Autodesk Inventor part; units mm, degrees
ref_plane "YZ Plane" through (0, 0, 0) normal (1, 0, 0) x (0, 1, 0)
ref_plane "XZ Plane" through (0, 0, 0) normal (0, 1, 0) x (-1, 0, 0)
ref_plane "XY Plane" through (0, 0, 0) normal (0, 0, 1) x (1, 0, 0)
sketch "Náčrt1" plane through (0, 0, 0) normal (0, 0, 1) x (1, 0, 0)
  line L0 (-9.5, 7.7937) -> (-9.5, -1.7063)
  line L1 (-9.5, -1.7063) -> (9.5, -1.7063)
  line L2 (9.5, -1.7063) -> (9.5, 7.7937)
  line L3 (9.5, 7.7937) -> (10, 7.7937)
  line L4 (10, 7.7937) -> (10, -2.2063)
  line L5 (10, -2.2063) -> (-10, -2.2063)
  line L6 (-10, -2.2063) -> (-10, 7.7937)
  line L7 (-10, 7.7937) -> (-9.5, 7.7937)
  point P0 (0, 0)
  point P1 (9.5, 3.0437)
  point P2 (-9.75, 7.7937)
  point P3 (9.75, 7.7937)
  dimension "d0" = 10
  dimension "d1" = 10
  dimension "d2" = 0.5
  dimension "d3" = 0.5
  dimension "d4" = 0.5
  dimension "d5" = 10
  dimension "d6" = 10
extrude "Vysunutí1" add sketch "Náčrt1" along normal blind 10
sketch "Náčrt2" plane through (10, -2.2063, 0) normal (1, 0, 0) x (0, 0, -1)
  circle A0 centre (-5, 5) radius 2
  line L0 (0, 0) -> (0, 10)
  point P0 (0, 2.2063)
  point P1 (0, 5)
  dimension "d9" = 4
  dimension "d10" = 5
extrude "Vysunutí2" cut sketch "Náčrt2" against normal through all
pattern_linear "Obdélníkové pole1" count 10 spacing 10 along (0, 0, 1) of "Vysunutí2"
sketch "Náčrt3" plane through (-9.5, -1.7063, 0) normal (0, 1, 0) x (1, 0, 0)
  circle A0 centre (4.5, -5) radius 2
  line L0 (19, -10) -> (0, -10)
  line L1 (-0.5, 0) -> (-0.5, -10)
  point P0 (9.5, 0)
  dimension "d16" = 4
  dimension "d17" = 5
  dimension "d18" = 5
extrude "Vysunutí3" cut sketch "Náčrt3" against normal through all
pattern_linear "Obdélníkové pole2" count 10 spacing 10 along (0, 0, -1) count 5 spacing 10 along (1, 0, 0) of "Vysunutí3"
sketch "Náčrt4" plane through (10, -2.2063, 0) normal (1, 0, 0) x (0, 0, -1)
  arc A0 (0, 5) -> (-10, 5) centre (-5, 5) ccw
  line L0 (0, 0) -> (0, 10)
  line L1 (0, 0) -> (-10, 0)
  line L2 (0, 10) -> (-10, 10)
  line L3 (-10, 10) -> (0, 10)
  line L4 (0, 10) -> (0, 5)
  line L5 (0, 10) -> (0, 0.5)
  line L6 (-10, 10) -> (-10, 0.5)
  line L7 (-10, 5) -> (-10, 10)
  point P0 (0, 2.2063)
  point P1 (-5, 10)
  dimension "d27" = 10
  dimension "d28" = 5
  dimension "d29" = 5
extrude "Vysunutí4" cut sketch "Náčrt4" against normal through all
fillet "Zaoblení1" radius 0.5 2 edges at (10, -2.2063, 5) (9.5, -1.7063, 5)
fillet "Zaoblení2" radius 0.5 2 edges at (-10, -2.2063, 5) (-9.5, -1.7063, 5)
properties part number "4031"
Can you work these out from the model? Positions are in its coordinate system, mm. A direction names the side the tool comes from. Coordinates: 2 decimals unless noted, no trailing zeros. Order: outer loops, then holes, each group sorted by start corner. A loop starts at its lowest first (then second) coordinate and runs counter-clockwise, first axis right, second up. Notation, with made-up numbers: M 72,80.25 L 125,80.25 A27 ccw 125,113.25 Z; hole C -3.75,56.25 d8. An arc over 180 degrees is marked long. Write item = value, one per line.
(1) Suppose I cut it at B-B on x = 5. Please give me the cut outline in (y, z).
Results are:
outline = M -2.21,0 L -1.71,0 L -1.71,3 L -2.21,3 Z; M -2.21,7 L -1.71,7 L -1.71,10 L -2.21,10 Z
(2) For pin 1 Ø3 at (x, z) = (-5, 5) entering from -Y, with a flat end and sliding along its axis, tell me the tip position at first contact or that it passes through.
Results are:
pin_1 = through
(3) For faces 1 (the face through (0, -1.706, 5)), 2 (the face through (0, -2, 10)), which set-ups out of +Z, -Z, +X, -X, +Y, -Y let a thin tool reach every point of the face, with its end or its side?
Results are:
face_1 = +Z, -Z, +Y
face_2 = +Z, +X, -X, +Y, -Y
(4) Suppose I cut it at D-D on z = 1.75. Please give me the cut outline in (x, y).
Results are:
outline = M -10,-1.71 A0.5 ccw -9.5,-2.21 L 9.5,-2.21 A0.5 ccw 10,-1.71 L 10,6.59 L 9.5,6.59 L 9.5,-1.21 A0.5 cw 9,-1.71 L -9,-1.71 A0.5 cw -9.5,-1.21 L -9.5,6.59 L -10,6.59 Z
(5) Suppose I cut it at A-A on z = 5. Please give me the cut outline in (x, y), plus the area to 3 significant figures.
Results are:
outline = M -10,-1.71 A0.5 ccw -9.5,-2.21 L -7,-2.21 L -7,-1.71 L -9,-1.71 A0.5 cw -9.5,-1.21 L -9.5,0.79 L -10,0.79 Z; M -10,4.79 L -9.5,4.79 L -9.5,7.79 L -10,7.79 Z; M -3,-2.21 L 3,-2.21 L 3,-1.71 L -3,-1.71 Z; M 7,-2.21 L 9.5,-2.21 A0.5 ccw 10,-1.71 L 10,0.79 L 9.5,0.79 L 9.5,-1.21 A0.5 cw 9,-1.71 L 7,-1.71 Z; M 9.5,4.79 L 10,4.79 L 10,7.79 L 9.5,7.79 Z
area = 11.5 mm2
(6) If we mould it in two halves opening along Z, with no side actions, what happens to faces 3 (the face through (9.5, 3.2, 2.7)), 4 (the face through (-9.747, 7.792, 4.89)), 5 (the face through (3.4, -2, 6.2))? For each: pulls with the +Z half, pulls with the -Z half, needs draft (parallel to the pull), parting line crosses it, or undercut.
Results are:
face_3 = needs draft
face_4 = parting line crosses it
face_5 = undercut
(7) Suppose I cut it at C-C on y = 5.5. Please give me the cut outline in (x, z).
Results are:
outline = M -10,0.8 L -9.5,0.8 L -9.5,9.2 L -10,9.2 Z; M 9.5,0.8 L 10,0.8 L 10,9.2 L 9.5,9.2 Z
(8) I need wall thicknesses on line 1 along X through (y, z) = (-1.75, 5); line 2 along Z through (x, y) = (-5, -1.9); line 3 along X through (y, z) = (2.5, 1). Which ranges of each line are inside material? Lowest first, please. Write a range as [from, to].
Results are:
line_1 = [-10, -7], [-3, 3], [7, 10]
line_2 = [0, 3], [7, 10]
line_3 = [-10, -9.5], [9.5, 10]
